from build123d import *

# Parameters (mm, degrees)
SKETCH_1_W          = 3
SKETCH_1_H          = 2.5
SKETCH_2_W          = 53.705080546
SKETCH_2_H          = 2
CUT_EXTRUDE_1_DEPTH = 1.5


with BuildPart() as part:
    # 草图1 → 旋转1 (revolve)
    with BuildSketch(Plane.XY, mode=Mode.PRIVATE) as revolve_1_sk:
        with Locations((6, -3.214249787)):
            Rectangle(SKETCH_1_W, SKETCH_1_H)
    revolve(revolve_1_sk.sketch.rotate(Axis((0, 56.260842627, 0), (0, -1, 0)), 90), axis=Axis((0, 56.260842627, 0), (0, -1, 0)))  # turned: the seam where the file's is

    # 草图2 → 切除-拉伸1 (cut)
    with BuildSketch(Plane(origin=(0, -1.964249787, 0), x_dir=(1, 0, 0), z_dir=(0, 1, 0))):
        Rectangle(SKETCH_2_W, SKETCH_2_H)
    extrude(amount=-CUT_EXTRUDE_1_DEPTH, mode=Mode.SUBTRACT)


solid = part.part
Read the model definition and answer for the solid it produces. Units are mm, in the model's axes. A direction names the side the tool comes from. Coordinates: 2 decimals unless noted, no trailing zeros. Order: outer loops, then holes, each group sorted by start corner. A loop starts at its lowest first (then second) coordinate and runs counter-clockwise, first axis right, second up. Notation, with made-up numbers: M 20.5,70.5 L 58.5,70.5 A20 ccw 58.5,101.5 Z; hole C 55,-13 d11. An arc over 180 degrees is marked long. Put each result on its own line as item: value. Start each with the question number.
Item 1: Section C-C, the plane y = -3.75 is taken. Determine the outline of the cut face in (x, z).
Item 2: For faces 1 (the face through (0, -1.964, -5)), 2 (the face through (-6, -3, 1)), determine the directions among +Z, -Z, +X, -X, +Y, -Y from which every point of the face is accessible in a straight line to the end or side of a thin tool.
Item 3: The mould has two halves that part along Z. Classify faces 3 (the face through (6, -3, -1)), 4 (the face through (0, -1.964, 5)), 5 (the face through (7.32, -3.2, -1.63)): +Z half, -Z half, draft (parallel to the pull), parting line (faces both ways), or undercut.
Item 4: Given pin 1 Ø1.2 at (x, y) = (5.5, -2.5) entering from +Z; pin 2 Ø1 at (x, z) = (-6.5, 0) entering from +Y; pin 3 Ø1.2 at (x, y) = (-6.5, -2.5) entering from +Z, each flat-ended and moving along its own axis, determine where each tip first touches the part or whether it passes through.
Item 5: Section B-B, the plane z = 0 is taken. Determine the outline of the cut face in (x, y), plus the area to 3 significant figures.
Item 6: Section A-A, the plane x = 0 is taken. Determine the outline of the cut face in (y, z).
Item 7: Consider probe 1 along Z at (x, y) = (1, -2.7); probe 2 along X at (y, z) = (-3.9, 0); probe 3 along X at (y, z) = (-4.3, 0.75). Determine where each line is inside the solid, lowest interval first. Write a range as [from, to].
Item 8: Section D-D, the plane z = 6.5 is taken. Determine the outline of the cut face in (x, y).
Computed:
1. outline: C 0,0 d15; hole C 0,0 d9
2. face 1: +Z, -Z, +X, -X, +Y
2. face 2: +X, -X, +Y
3. face 3: undercut
3. face 4: draft
3. face 5: parting line
4. pin 1: stops at z = 5.68
4. pin 2: stops at y = -3.46
4. pin 3: stops at z = 4.63
5. outline: M -7.5,-4.46 L -4.5,-4.46 L -4.5,-3.46 L -7.5,-3.46 Z; M 4.5,-4.46 L 7.5,-4.46 L 7.5,-3.46 L 4.5,-3.46 Z
5. area: 6.00 mm2
6. outline: M -4.46,-7.5 L -1.96,-7.5 L -1.96,-4.5 L -4.46,-4.5 Z; M -4.46,4.5 L -1.96,4.5 L -1.96,7.5 L -4.46,7.5 Z
7. probe 1: z = [-7.43, -4.39], [4.39, 7.43]
7. probe 2: x = [-7.5, -4.5], [4.5, 7.5]
7. probe 3: x = [-7.46, -4.44], [4.44, 7.46]
8. outline: M -3.74,-4.46 L 3.74,-4.46 L 3.74,-1.96 L -3.74,-1.96 Z
